The listing builds one solid part. Answer for the finished solid, in the listing's coordinates (mm). Face numbers are marked on the shaded views. A direction names the side the tool comes from. Give positions to 0.01 mm unless a question says otherwise; leave off trailing zeros. Write each loop counter-clockwise with the first axis right and the second up, starting at its lowest first coordinate (ties: lowest second). Pieces come first, ordered by that corner, then holes.
```python
from build123d import *

# Parameters (mm, degrees)
SKETCH2_W           = 5
SKETCH2_H           = 7
BOSS_EXTRUDE1_DEPTH = 40
SKETCH3_R           = 2.05
CUT_EXTRUDE2_DEPTH  = 40
BOSS_EXTRUDE2_DEPTH = 40
SKETCH7_W           = 4.5
SKETCH7_H           = 2
CUT_EXTRUDE3_DEPTH  = 87.11081163
SKETCH8_W           = 1
SKETCH8_H           = 2
CUT_EXTRUDE4_DEPTH  = 5
BOSS_EXTRUDE3_DEPTH = 2
SKETCH10_W          = 2.5
SKETCH10_H          = 2
CUT_EXTRUDE5_DEPTH  = 11
BOSS_EXTRUDE4_DEPTH = 4
BOSS_EXTRUDE7_DEPTH = 4
BOSS_EXTRUDE8_DEPTH = 19
SKETCH17_R          = 2
CUT_EXTRUDE7_DEPTH  = 19
SKETCH18_W          = 2.5
SKETCH18_H          = 2
CUT_EXTRUDE8_DEPTH  = 2.5
SKETCH19_W          = 2.5
SKETCH19_H          = 2
CUT_EXTRUDE9_DEPTH  = 19.5
SKETCH20_W          = 2.3
SKETCH20_H          = 2
CUT_EXTRUDE10_DEPTH = 2.5
SKETCH21_W          = 2.5
SKETCH21_H          = 74.8
CUT_EXTRUDE11_DEPTH = 2.5


with BuildPart() as part:
    # Sketch2 → Boss-Extrude1 (new body)
    with BuildSketch(Plane(origin=(0, 0, 0), x_dir=(1, 0, 0), z_dir=(0, 1, 0))):
        Polygon((11.100217707, -10.156419986), (7.442255773, 6.343580014), (7.442255773, 1.343580014), (3.429331515, 1.343580014), (5.978820135, -10.156419986), align=None)
        Polygon((7.442255773, 6.343580014), (-10.583592744, 6.343580014), (-5.702112708, 5.261381945), (-6.570668485, 1.343580014), (3.429331515, 1.343580014), (2.560775738, 5.261381945), align=None)
        Polygon((-10.583592744, 1.343580014), (-10.583592744, 6.343580014), (-14.241554677, -10.156419986), (-9.120157106, -10.156419986), (-6.570668485, 1.343580014), align=None)
        Polygon((7.442255773, 1.343580014), (7.442255773, 6.343580014), (2.560775738, 5.261381945), (3.429331515, 1.343580014), align=None)
        Polygon((-5.702112708, 5.261381945), (-10.583592744, 6.343580014), (-10.583592744, 1.343580014), (-6.570668485, 1.343580014), align=None)
        Polygon((-9.360074642, -11.238618055), (-14.241554677, -10.156419986), (-14.241554677, -15.156419986), (-9.241554677, -15.156419986), (-4.241554677, -15.156419986), (-4.241554677, -10.156419986), (-9.120157106, -10.156419986), align=None)
        Polygon((-9.120157106, -10.156419986), (-14.241554677, -10.156419986), (-9.360074642, -11.238618055), align=None)
        Polygon((6.218737671, -11.238618055), (11.100217707, -10.156419986), (5.978820135, -10.156419986), align=None)
        Polygon((11.100217707, -15.156419986), (11.100217707, -10.156419986), (6.218737671, -11.238618055), (5.978820135, -10.156419986), (1.100217707, -10.156419986), (1.100217707, -15.156419986), (6.100217707, -15.156419986), align=None)
        with Locations((3.600217707, -18.656419986)):
            Rectangle(SKETCH2_W, SKETCH2_H)
        with Locations((-6.741554677, -18.656419986)):
            Rectangle(SKETCH2_W, SKETCH2_H)
    extrude(amount=BOSS_EXTRUDE1_DEPTH)

    # Sketch3 → Cut-Extrude2 (cut)
    with BuildSketch(Plane.ZY.offset(9.241554677)):
        with Locations((18.656419986, 33)):
            Circle(SKETCH3_R)
        with Locations((18.656419986, 7)):
            Circle(SKETCH3_R)
    extrude(amount=-CUT_EXTRUDE2_DEPTH, mode=Mode.SUBTRACT)

    # Sketch4 → Boss-Extrude2 (add)
    with BuildSketch(Plane(origin=(0, 40, 0), x_dir=(1, 0, 0), z_dir=(0, 1, 0))):
        Polygon((-4.241554677, -10.156419986), (-9.120157106, -10.156419986), (-6.570668485, 1.343580014), (3.429331515, 1.343580014), (5.978820135, -10.156419986), (1.100217707, -10.156419986), (1.100217707, -15.156419986), (6.100217707, -15.156419986), (11.100217707, -15.156419986), (11.100217707, -10.156419986), (7.442255773, 6.343580014), (-10.583592744, 6.343580014), (-14.241554677, -10.156419986), (-14.241554677, -15.156419986), (-9.241554677, -15.156419986), (-4.241554677, -15.156419986), align=None)
    extrude(amount=BOSS_EXTRUDE2_DEPTH)

    # Sketch7 → Cut-Extrude3 (cut, through all)
    with BuildSketch(Plane(origin=(0, 0, -6.343580014), x_dir=(-1, 0, 0), z_dir=(0, 0, -1))):
        with Locations((1.567744227, 4.2)):
            Rectangle(SKETCH7_W, SKETCH7_H)
    extrude(amount=-CUT_EXTRUDE3_DEPTH, mode=Mode.SUBTRACT)

    # Sketch8 → Cut-Extrude4 (cut)
    with BuildSketch(Plane(origin=(0, 0, 10.156419986), x_dir=(-1, 0, 0), z_dir=(0, 0, -1))):
        with Locations((4.741554677, 4.2)):
            Rectangle(SKETCH8_W, SKETCH8_H)
    extrude(amount=-CUT_EXTRUDE4_DEPTH, mode=Mode.SUBTRACT)

    # Sketch9 → Boss-Extrude3 (add)
    with BuildSketch(Plane(origin=(0, 80, 0), x_dir=(1, 0, 0), z_dir=(0, 1, 0))):
        Polygon((1.100217707, -10.156419986), (1.100217707, -12.156419986), (8.470768489, -12.156419986), (5.034501218, 3.343580014), (-8.175838189, 3.343580014), (-11.61210546, -12.156419986), (-4.241554677, -12.156419986), (-4.241554677, -10.156419986), (-9.120157106, -10.156419986), (-6.570668485, 1.343580014), (3.429331515, 1.343580014), (5.978820135, -10.156419986), align=None)
    extrude(amount=BOSS_EXTRUDE3_DEPTH)

    # Sketch10 → Cut-Extrude5 (cut)
    with BuildSketch(Plane(origin=(-5.241554677, 0, 0), x_dir=(0, 0, -1), z_dir=(1, 0, 0))):
        with Locations((-13.906419986, 4.2)):
            Rectangle(SKETCH10_W, SKETCH10_H)
    extrude(amount=-CUT_EXTRUDE5_DEPTH, mode=Mode.SUBTRACT)

    # Sketch11 → Boss-Extrude4 (add)
    with BuildSketch(Plane.XY.offset(15.156419986)):
        Polygon((11.100217707, 54.293335879), (29.100217707, 80), (11.100217707, 80), align=None)
        Polygon((-14.241554677, 54.293335879), (-32.241554677, 80), (-14.241554677, 80), align=None)
    extrude(amount=-BOSS_EXTRUDE4_DEPTH)

    # Sketch15 → Boss-Extrude7 (add)
    with BuildSketch(Plane(origin=(0, 0, -6.343580014), x_dir=(-1, 0, 0), z_dir=(0, 0, -1))):
        Polygon((-7.442255773, 80), (-7.442255773, 49.080595654), (-29.092255773, 80), align=None)
        Polygon((10.583592744, 80), (10.583592744, 49.080595654), (32.233592744, 80), align=None)
    extrude(amount=-BOSS_EXTRUDE7_DEPTH)

    # Sketch16 → Boss-Extrude8 (add)
    with BuildSketch(Plane(origin=(0, 0, -6.343580014), x_dir=(-1, 0, 0), z_dir=(0, 0, -1))):
        Polygon((32.233592744, 80), (29.432762591, 76), (10.233592744, 76), (10.233592744, 80), align=None)
        Polygon((-29.092255773, 80), (-26.29142562, 76), (-7.092255773, 76), (-7.092255773, 80), align=None)
    extrude(amount=-BOSS_EXTRUDE8_DEPTH)

    # Sketch17 → Cut-Extrude7 (cut)
    with BuildSketch(Plane(origin=(0, 76, 0), x_dir=(-1, 0, 0), z_dir=(0, -1, 0))):
        with Locations(Location((-19.01946661, -4.406419986, 0), (0, 0, 90))):
            Circle(SKETCH17_R)
        with Locations(Location((18.980533391, -4.406419986, 0), (0, 0, 90))):
            Circle(SKETCH17_R)
    extrude(amount=-CUT_EXTRUDE7_DEPTH, mode=Mode.SUBTRACT)

    # Sketch18 → Cut-Extrude8 (cut)
    with BuildSketch(Plane.XY.offset(12.656419986)):
        with Locations((-12.991554677, 4.2)):
            Rectangle(SKETCH18_W, SKETCH18_H)
    extrude(amount=-CUT_EXTRUDE8_DEPTH, mode=Mode.SUBTRACT)

    # Sketch19 → Cut-Extrude9 (cut, along a direction that is not the sketch's normal)
    with BuildSketch(Plane.XY.offset(10.156419986)):
        with Locations((-12.991554677, 4.2)):
            Rectangle(SKETCH19_W, SKETCH19_H)
    extrude(amount=-CUT_EXTRUDE9_DEPTH, dir=(-0.2164396139381068, 0, 0.9762960071199325), mode=Mode.SUBTRACT)

    # Sketch20 → Cut-Extrude10 (cut, along a direction that is not the sketch's normal)
    with BuildSketch(Plane(origin=(-9.045364277, 0, -2.005308982), x_dir=(-0.2164396139381068, 0, 0.9762960071199326), z_dir=(-0.9762960071199326, 0, -0.2164396139381068))):
        with Locations((-3.293602146, 4.2)):
            Rectangle(SKETCH20_W, SKETCH20_H)
    extrude(amount=-CUT_EXTRUDE10_DEPTH, dir=(-1, 0, 0), mode=Mode.SUBTRACT)

    # Sketch21 → Cut-Extrude11 (cut)
    with BuildSketch(Plane(origin=(0, 0, -6.343580014), x_dir=(-1, 0, 0), z_dir=(0, 0, -1))):
        with Locations((1.567744227, 42.6)):
            Rectangle(SKETCH21_W, SKETCH21_H)
        with Locations((6.833592744, 42.6)):
            Rectangle(SKETCH21_W, SKETCH21_H)
    extrude(amount=-CUT_EXTRUDE11_DEPTH, mode=Mode.SUBTRACT)


solid = part.part
```
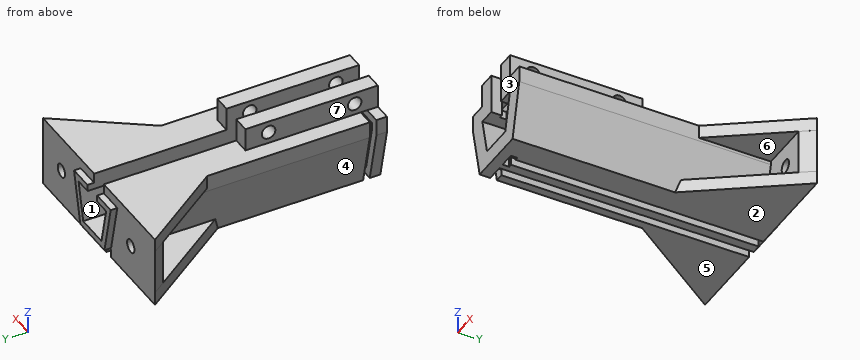
Item 1: Determine the mould class of the marked faces 1, 2 and 3 for opening direction Z: pulls with the +Z half, pulls with the -Z half, needs draft (parallel to the pull), parting line crosses it, or undercut.
Conclusion:
face 1: undercut
face 2: pulls with the -Z half
face 3: needs draft
Item 2: Which of the six approach directions +Z, -Z, +X, -X, +Y, -Y give full straight-line access (tool end or side, diameter ignored) to the marked faces 4, 5, 6 and 7?
Conclusion:
face 4: -X, -Y
face 5: -Z, +X, -X, +Y, -Y
face 6: +X, -Y
face 7: +Z, -X, +Y, -Y
Item 3: A cutting plane is placed at C-C, the plane z = 1.5. Give the vertices of the cut face in (x, y), plus the area to 3 significant figures.
Conclusion:
outline: (-32.23, 80) - (-29.43, 76) - (-12.32, 76) - (-12.32, 5.2) - (-9.82, 5.2) - (-9.82, 3.2) - (-12.32, 3.2) - (-12.32, 0) - (-7.2, 0) - (-7.2, 82) - (-9.25, 82) - (-9.25, 80) - close; (4.06, 0) - (9.18, 0) - (9.18, 76) - (26.29, 76) - (29.09, 80) - (6.11, 80) - (6.11, 82) - (4.06, 82) - close
area: 971 mm2
Item 4: A cutting plane is placed at D-D, the plane x = -27. Give the vertices of the cut face in (y, z), plus the area to 3 significant figures.
Conclusion:
outline: (72.51, 11.16) - (76, 11.16) - (76, -2.34) - (72.53, -2.34) - (72.53, -6.34) - (80, -6.34) - (80, 15.16) - (72.51, 15.16) - close
area: 114 mm2
Item 5: A cutting plane is placed at A-A, the plane y = 7. Count the separate pieces of the cut face and the enclosed holes in it, plus the area to 3 significant figures.
Conclusion:
separate pieces: 3
enclosed holes: 0
area: 330 mm2
Item 6: Each of these flat-tipped pins is pushed along its axis until it touches: P1, Ø6, axis at y = 21.5, z = 15.5, coming from the -X side; P2, Ø1, axis at x = 7.5, z = -1.5, coming from the +Y side; P3, Ø3.5, axis at y = 7, z = 18.66, coming from the -X side; P4, Ø9, axis at x = 16, y = 64.5, coming from the +Z side. Where does it stop, or does it pass through?
Conclusion:
P1: stops at x = -14.24
P2: stops at y = 80
P3: passes through
P4: stops at z = 15.16
Item 7: A cutting plane is placed at B-B, the plane y = 21.5. Give the vertices of the cut face in (x, z).
Conclusion:
outline: (-14.24, 10.16) - (-10.58, -6.34) - (-8.08, -6.34) - (-8.08, -3.84) - (-5.58, -3.84) - (-5.58, -6.34) - (-2.82, -6.34) - (-2.82, -3.84) - (-0.32, -3.84) - (-0.32, -6.34) - (7.44, -6.34) - (11.1, 10.16) - (11.1, 15.16) - (6.1, 15.16) - (6.1, 22.16) - (1.1, 22.16) - (1.1, 10.16) - (5.98, 10.16) - (3.43, -1.34) - (-6.57, -1.34) - (-9.12, 10.16) - (-4.24, 10.16) - (-4.24, 22.16) - (-9.24, 22.16) - (-9.24, 15.16) - (-14.24, 15.16) - close
Item 8: Consider probe 1 along X at (y, z) = (67, 11); probe 2 along Y at (x, z) = (26, -2.25); probe 3 along X at (y, z) = (45.5, -4.75). Determine where each line is inside the solid, lowest interval first.
Conclusion:
probe 1: x = -14.24 to -4.24, 1.1 to 11.1
probe 2: y = 76 to 80
probe 3: x = -10.94 to -8.08, -5.58 to -2.82, -0.32 to 7.8
